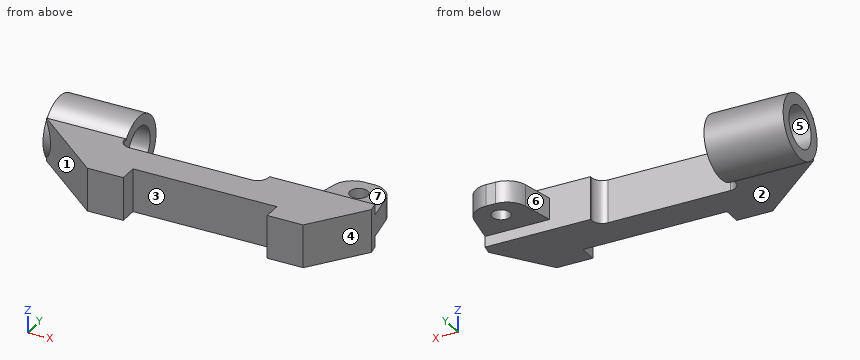
Autodesk Inventor part; units mm, degrees
ref_plane "YZ Plane" through (0, 0, 0) normal (1, 0, 0) x (0, 1, 0)
ref_plane "XZ Plane" through (0, 0, 0) normal (0, 1, 0) x (-1, 0, 0)
ref_plane "XY Plane" through (0, 0, 0) normal (0, 0, 1) x (1, 0, 0)
sketch "Szkic1" plane through (0, 0, 0) normal (0, 0, 1) x (1, 0, 0)
  line L0 (0, 5) -> (0, 0)
  line L1 (0, 0) -> (10, 0)
  line L2 (0, 5) -> (-40, 5)
  line L3 (-40, 5) -> (-40, 0)
  line L4 (-40, 0) -> (-50, 0)
  line L5 (-50, 0) -> (-70.7267, 17.3918)
  line L6 (-70.7267, 17.3918) -> (-48.7267, 17.3918)
  line L7 (-48.7267, 17.3918) -> (-48.7267, 13.8918)
  line L8 (-48.7267, 13.8918) -> (-8.7267, 13.8918)
  line L9 (-8.7267, 13.8918) -> (-8.7267, 17.3918)
  line L10 (-8.7267, 17.3918) -> (2.6733, 17.3918)
  line L11 (2.6733, 17.3918) -> (5.7412, 30.6804)
  line L12 (18.2412, 30.6804) -> (5.7412, 30.6804)
  line L13 (10, 0) -> (21.0625, 14.6804)
  line L14 (18.2412, 30.6804) -> (21.0625, 14.6804)
  circle A0 centre (11.9912, 25.0804) radius 2.5
  line L15 (2.6733, 17.3918) -> (20.5844, 17.3918)
  point P0 (11.9912, 30.6804)
  dimension "d0" = 10
  dimension "d1" = 40
  dimension "d2" = 10
  dimension "d3" = 22
  dimension "d4" = 3.5
  dimension "d5" = 40
  dimension "d6" = 11.4
  dimension "d7" = 103
  dimension "d8" = 12.5
  dimension "d9" = 127
  dimension "d10" = 16
  dimension "d11" = 5
  dimension "d12" = 133
  dimension "d13" = 5
  dimension "d14" = 5.6
extrude "Wyciągnięcie proste1" add sketch "Szkic1" along normal mid plane 12 contours L2 L3 L4 L5 L6 L7 L8 L9 L10 L15 L14 L13 L1 L0
extrude "Wyciągnięcie proste2" add sketch "Szkic1" along normal mid plane 6 contours L15 L11 L12 L14
fillet "Zaokrąglenie1" radius 3 1 edges at (-48.7267, 13.8918, 0)
fillet "Zaokrąglenie2" radius 3 1 edges at (-8.7267, 13.8918, 0)
fillet "Zaokrąglenie3" radius 6 1 edges at (18.2412, 30.6804, 0)
fillet "Zaokrąglenie4" radius 6 1 edges at (5.7412, 30.6804, 0)
sketch "Szkic3" plane through (-48.7267, 17.3918, 6) normal (1, 0, 0) x (0, 0, -1)
  line L0 (12, 0) -> (0, 0)
  circle A0 centre (6, 7) radius 8.75
  circle A1 centre (6, 7) radius 5.75
  point P0 (6, -17.3918)
  dimension "d39" = 17.5
  dimension "d40" = 11.5
extrude "Wyciągnięcie proste3" add sketch "Szkic3" against normal blind 22 contours A0 L0 | L0 A0 | A1
extrude "Wyciągnięcie proste4" cut sketch "Szkic3" against normal blind 22 contours A1
properties material "Stal"
Verification items for the finished model (mm, model axes). Face numbers are marked on the shaded views. A direction names the side the tool comes from. Coordinates: 2 decimals unless noted, no trailing zeros. Loops run counter-clockwise (first coordinate to the right, second up) from the corner with the lowest first, then second, coordinate; pieces in that order, holes last. Notation, with made-up numbers: (-7.75, -28.5) -> (46.25, -28.5) arc R24 ccw to (46.25, -7.5) -> close; hole circle Ø4 at (-28, -31). An arc over 180 degrees is marked (long way). Write each question's results on one line, items separated by ' | '.
Item 1: Section check A-A, the plane z = -1. Enter the section's corners in (x, y).
Found:
outline: (-70.73, 15.7) -> (-68.71, 15.7) -> (-50, 0) -> (-40, 0) -> (-40, 5) -> (0, 5) -> (0, 0) -> (10, 0) -> (21.06, 14.68) -> (19.12, 25.72) arc R6 ccw to (13.21, 30.68) -> (10.51, 30.68) arc R6 ccw to (4.67, 26.03) -> (2.67, 17.39) -> (-8.73, 17.39) -> (-8.73, 16.89) arc R3 cw to (-11.73, 13.89) -> (-45.73, 13.89) arc R3 cw to (-48.73, 16.89) -> (-48.73, 18.73) -> (-70.73, 18.73) -> close; (-70.73, 30.05) -> (-48.73, 30.05) -> (-48.73, 33.08) -> (-70.73, 33.08) -> close; hole circle Ø5 at (11.99, 25.08)
Item 2: Tool access check on the marked faces 5, 6 and 7. Record the directions out of +Z, -Z, +X, -X, +Y, -Y that give a thin tool (end or side, any length) a straight path to the whole face; none if there is none.
Found:
face 5: -X | face 6: +Z, -Z, +Y | face 7: +Z, +X, +Y
Item 3: Material ranges on L1, parallel to Y at x = -7, z = 0; L2, parallel to Y at x = -49.5, z = -2; L3, parallel to Y at x = -51.5, z = 2.75, recorded low to high.
Found:
L1: y = 5 to 17.39 | L2: y = 0 to 19, 29.78 to 32.91 | L3: y = 1.26 to 19.34, 29.44 to 32.7
Item 4: Section check D-D, the plane y = 10. Enter the section's corners in (x, z).
Found:
outline: (-61.92, -6) -> (17.54, -6) -> (17.54, 6) -> (-61.92, 6) -> close
Item 5: Section check C-C, the plane x = 7. Enter the section's corners in (y, z), plus the area to 3 significant figures.
Found:
outline: (0, -6) -> (17.39, -6) -> (17.39, -3) -> (29.54, -3) -> (29.54, 3) -> (17.39, 3) -> (17.39, 6) -> (0, 6) -> close | area: 282 mm2
Item 6: Mould release check, pull along X, two halves, no side actions. Record for the marked faces 1, 2, 3 and 4: +X half, -X half, draft (parallel to the pull), parting line (faces both ways), or undercut.
Found:
face 1: -X half | face 2: draft | face 3: undercut | face 4: +X half
Item 7: Gauge pin test, flat ends, axial feed: pin 1 (1.5 mm diameter, centred on x = -34.5, z = -0.5, fed in from +Y); pin 2 (5 mm diameter, centred on x = -32, y = 9.5, fed in from +Z); pin 3 (0.8 mm diameter, centred on x = 12, z = 0, fed in from +Y); pin 4 (6 mm diameter, centred on x = -41, z = -0.5, fed in from -Y). Record the tip position at first contact, or that the pin passes through.
Found:
pin 1: stops at y = 13.89 | pin 2: stops at z = 6 | pin 3: stops at y = 30.68 | pin 4: stops at y = 0
Item 8: Section check B-B, the plane x = -54. Enter the section's corners in (y, z).
Found:
outline: (3.36, -6) -> (17.39, -6) -> (17.39, -5.25) arc R8.75 ccw (long way) to (17.39, 5.25) -> (17.39, 6) -> (3.36, 6) -> close; hole circle Ø11.5 at (24.39, 0)
